from build123d import *

# Parameters (mm, degrees)
PAD004_DEPTH          = 7
CLONE_PLACEMENT_ANGLE = -90
SKETCH009_W           = 14
SKETCH009_H           = 14
PAD003_DEPTH          = 3
POCKET006_DEPTH       = 2
SKETCH011_R           = 0.9
POCKET007_DEPTH       = 1.001


with BuildPart() as array:
    # Sketch012 → Pad004 (new body, symmetric)
    with BuildSketch(Plane.YZ):
        Polygon((-8, 0), (-8, 3.3), (-5.5, 3.3), (-5.5, 7.5), (-3.4, 7.5), (-3.4, 6.9), (-4.2, 6.1), (-4.2, 3.3), (-1.9, 3.3), (-1.9, 2.3), (-0.7, 2.3), (-0.7, 3.3), (4.2, 3.3), (4.2, 6.1), (3.4, 6.9), (3.4, 7.5), (5.5, 7.5), (5.5, 3.3), (8, 3.3), (8, 0), align=None)
    extrude(amount=PAD004_DEPTH, both=True)


with BuildPart() as array_1:
    # Clone placement: moved
    add(array.part.moved(Location((15, 0, 0))).rotate(Axis((15, 0, 0), (0, 0, 1)), CLONE_PLACEMENT_ANGLE))


with BuildPart() as obj1:
    # Sketch009 → Pad003 (new body)
    with BuildSketch(Plane.XY):
        Rectangle(SKETCH009_W, SKETCH009_H)
    extrude(amount=PAD003_DEPTH)

    # Sketch010 → Pocket006 (cut)
    with BuildSketch(Plane.XY.offset(3)):
        with BuildLine():
            Line((-3, 7), (-3, 4.963869))
            ThreePointArc((-3, 4.963869), (-5.8, 0), (-3, -4.963869))
            Line((-3, -7), (-3, -4.963869))
            Line((3, -7), (-3, -7))
            Line((3, -4.963869), (3, -7))
            ThreePointArc((3, -4.963869), (5.8, 0), (3, 4.963869))
            Line((3, 7), (3, 4.963869))
            Line((-3, 7), (3, 7))
        make_face()
    extrude(amount=-POCKET006_DEPTH, mode=Mode.SUBTRACT)

    # Sketch011 → Pocket007 (cut, through all)
    with BuildSketch(Plane.XY.offset(1)):
        Circle(SKETCH011_R)
    extrude(amount=-POCKET007_DEPTH, mode=Mode.SUBTRACT)


with BuildPart() as board_clamp_generic_fusion:
    # Clone008003 base: copy of obj1
    add(obj1.part)


with BuildPart() as board_clamp_generic_fusion_1:
    # Clone008003 placement: moved
    add(board_clamp_generic_fusion.part.moved(Location((30, 0, 0))))

    # Fusion: union Array, obj1
    add(array_1.part)
    add(obj1.part)


solid = board_clamp_generic_fusion_1.part
Can you work these out from the model? Positions are in its coordinate system, mm. A direction names the side the tool comes from. Round coordinates to 2 decimals unless told otherwise and drop trailing zeros. Write each loop counter-clockwise with the first axis right and the second up, starting at its lowest first coordinate (ties: lowest second). Pieces come first, ordered by that corner, then holes. Notation, with made-up numbers: (71, -28.5) -> (97, -28.5) arc R28 cw to (97, 9.5) -> close; hole circle Ø5 at (28.5, 40). An arc over 180 degrees is marked (long way). One line per question, with ' | ' between items. Start each with the question number.
1) Suppose I cut it at A-A on z = 6.5. Write out the boundary of the cut face in (x, y).
2) On a 3-axis mill with a long thin cutter (end or side, diameter ignored), from which of +Z, -Z, +X, -X, +Y, -Y can I reach the whole of each face in a straight line? I mean faces 4 (the flat face through (22, 0, 3.3)), 5 (the flat face through (8, 0, 3.3)), 6 (the flat face through (15, 7, 3)), 7 (the flat face through (15, -7, 3)), 8 (the flat face through (27, 6, 2)). Say none if no direction works.
3) I need wall thicknesses on line 1 (X direction, y = 5.5, z = 1.75); line 2 (X direction, y = -4.25, z = 4.5); line 3 (Y direction, x = 30, z = 0.5). Which ranges of each line are inside material? Lowest first, please. Write a range as [from, to].
4) If we mould it in two halves opening along X, with no side actions, what happens to faces 1 (the flat face through (9.5, 0, 5)), 2 (the flat face through (27, -6, 2)), 3 (the flat face through (6, 0, 3))? For each: released by +X, released by -X, zero draft, split by the parting line, or undercut.
5) Suppose I cut it at B-B on x = 0. Write out the boundary of the cut face in (y, z).
6) Suppose I cut it at D-D on y = 0. Count the separate pieces of the cut face and the enclosed holes in it, then the cut area to 3 significant figures.
7) I'm going to push flat-ended pins straight in: P1, Ø2, axis at x = 30, y = 0, coming from the +Z side; P2, Ø2, axis at x = 22, y = -2, coming from the +Z side; P3, Ø3, axis at x = 35, y = -2.5, coming from the +Z side. Where does each tip first touch, or does it pass through?
Return value:
1) outline: (9.5, -7) -> (11.2, -7) -> (11.2, 7) -> (9.5, 7) -> close; (18.8, -7) -> (20.5, -7) -> (20.5, 7) -> (18.8, 7) -> close
2) face 4: +Z, +X, +Y, -Y | face 5: +Z, -X, +Y, -Y | face 6: +Z, -Z, +X, -X, +Y | face 7: +Z, -Z, +X, -X, -Y | face 8: +Z, +Y, -Y
3) line 1: x = [-7, -3], [3, 27], [33, 37] | line 2: x = [9.5, 10.8], [19.2, 20.5] | line 3: y = [-7, -0.9], [0.9, 7]
4) face 1: released by -X | face 2: undercut | face 3: zero draft
5) outline: (-7, 0) -> (-0.9, 0) -> (-0.9, 1) -> (-7, 1) -> close; (0.9, 0) -> (7, 0) -> (7, 1) -> (0.9, 1) -> close
6) separate pieces: 3 | enclosed holes: 0 | area: 98.1 mm2
7) P1: stops at z = 1 | P2: stops at z = 3.3 | P3: stops at z = 3
